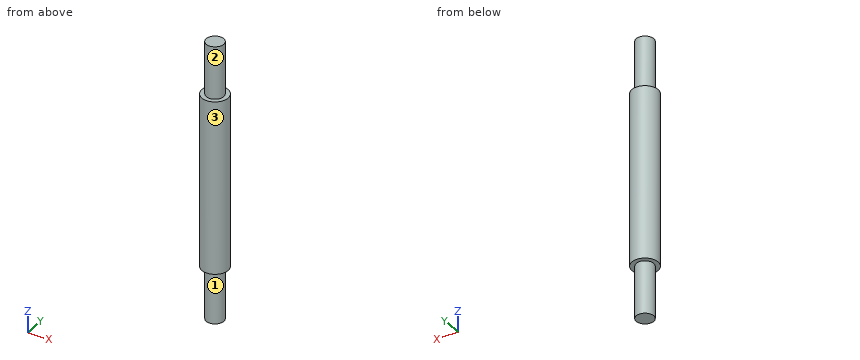
Autodesk Inventor part; units mm, degrees
ref_plane "BasePlane" through (-230.8476, -175.3438, -99) normal (0, 0, -1) x (0, 1, 0)
ref_plane "YZ Plane" through (0, 0, 0) normal (1, 0, 0) x (0, 1, 0)
ref_plane "XZ Plane" through (0, 0, 0) normal (0, 1, 0) x (-1, 0, 0)
sketch "Base" plane through (0, 0, 0) normal (0, 0, 1) x (1, 0, 0)
  line L0 (-3.5, 1.9365) -> (-3.5, -1.9365)
  line L1 (0, -5.6) -> (0, 5.6) construction
  circle A0 centre (0, 0) radius 4
  point P0 (-3.5, 0)
  dimension "d9" = 8
  dimension "d11" = 3.5
ref_plane "BasePlane" through (-230.8476, -175.3438, -99) normal (0, 0, -1) x (0, 1, 0)
extrude "BaseFeature" add sketch "Base" against normal up to surface (99 mm away)
sketch "Sketch4" plane through (0, 0, 0) normal (0, 0, 1) x (1, 0, 0)
  circle A0 centre (0, 0) radius 4
extrude "Extrusion4" add sketch "Sketch4" along normal blind 14
sketch "Sketch5" plane through (0, 0, -99) normal (0, 0, -1) x (0, 1, 0)
  circle A0 centre (0, 0) radius 4
  point P0 (0, 0)
extrude "Extrusion5" add sketch "Sketch5" along normal blind 14
ref_plane "StartPlane" through (-70.1743, -50.75, -10) normal (0, 0, -1) x (-0.0588, -0.9983, 0)
ref_plane "EndPlane" through (2.103, 3.913, -89) normal (0, 0, 1) x (-0.0671, 0.9977, 0)
sketch "Sketch6" plane through (-70.1743, -50.75, -10) normal (0, 0, -1) x (-0.0588, -0.9983, 0)
  circle A0 centre (-54.7868, -67.0701) radius 4.165
  circle A1 centre (-54.7868, -67.0701) radius 6
  point P0 (-54.7868, -67.0701)
  dimension "d16" = 12
extrude "Extrusion6" add sketch "Sketch6" along normal up to surface (79 mm away) contours A0 | A1
properties part number "LegKneeShaft"
Can you work these out from the model? Positions are in its coordinate system, mm. Face numbers are marked on the shaded views. A direction names the side the tool comes from. Round coordinates to 2 decimals unless told otherwise and drop trailing zeros. Write each loop counter-clockwise with the first axis right and the second up, starting at its lowest first coordinate (ties: lowest second). Pieces come first, ordered by that corner, then holes. Notation, with made-up numbers: M -40,1.25 L -5,1.25 A25 ccw -5,38.25 Z; hole C 21,34.5 d2. An arc over 180 degrees is marked long. Use a Markdown table: item, result.
Item 1: Which directions (+Z, -Z, +X, -X, +Y, -Y) give clear straight access to the entire face, cutting with the end or side of a thin tool? Please do the marked faces 1, 2 and 3.
Found:
| item | result |
|---|---|
| face 1 | -Z |
| face 2 | +Z |
| face 3 | +Z, -Z |
Item 2: For pin 1 Ø2 at (x, z) = (3.5, -0.5) entering from -Y, with a flat end and sliding along its axis, tell me the tip position at first contact or that it passes through.
Found:
| item | result |
|---|---|
| pin 1 | stops at y = -3.12 |
Item 3: If I drill on line 1 along Y through (x, z) = (0.25, -30); line 2 along Z through (x, y) = (-2.5, 5.25); line 3 along Y through (x, z) = (-4, -70), over which ranges is the centre line in solid material (lowest first)? Write a range as [from, to].
Found:
| item | result |
|---|---|
| line 1 | y = [-6, 5.99] |
| line 2 | z = [-89, -10] |
| line 3 | y = [-4.47, 4.47] |
Item 4: I want a section at A-A (z = -4). List the corners of the cut face in (x, y) for me, and give its area (3 significant figures).
Found:
| item | result |
|---|---|
| outline | C 0,0 d8 |
| area | 50.3 mm2 |
